```python
from build123d import *

# Parameters (mm, degrees)
SKETCH1_R                = 3.81
BOSS_EXTRUDE1_DEPTH      = 22.86
SKETCH2_R                = 3.81
BOSS_EXTRUDE2_DEPTH      = 3.81
BOSS_EXTRUDE2_DEPTH_BACK = 3.81
SKETCH4_R                = 2.54
CUT_EXTRUDE1_DEPTH       = 8.62
SKETCH5_R                = 3.302
CUT_EXTRUDE2_DEPTH       = 0.762
SKETCH6_R                = 3.302
CUT_EXTRUDE3_DEPTH       = 0.762


with BuildPart() as part:
    # Sketch1 → Boss-Extrude1 (new body)
    with BuildSketch(Plane.XY):
        with Locations((1.524, 0)):
            Circle(SKETCH1_R)
        with BuildLine():
            ThreePointArc((0, -0.762), (-0.762, 0), (0, 0.762))
            Line((0, 0.762), (0.762, 0.762))
            Line((0.762, 0.762), (0.762, 1.524))
            ThreePointArc((0.762, 1.524), (1.524, 2.286), (2.286, 1.524))
            Line((2.286, 1.524), (2.286, 0.762))
            Line((2.286, 0.762), (3.048, 0.762))
            ThreePointArc((3.048, 0.762), (3.81, 0), (3.048, -0.762))
            Line((3.048, -0.762), (2.286, -0.762))
            Line((2.286, -0.762), (2.286, -1.524))
            ThreePointArc((2.286, -1.524), (1.524, -2.286), (0.762, -1.524))
            Line((0.762, -1.524), (0.762, -0.762))
            Line((0.762, -0.762), (0, -0.762))
        make_face(mode=Mode.SUBTRACT)
    extrude(amount=BOSS_EXTRUDE1_DEPTH)

    # Sketch2 → Boss-Extrude2 (add, two sides)
    with BuildSketch(Plane(origin=(0, 0, 0), x_dir=(1, 0, 0), z_dir=(0, 1, 0))) as boss_extrude2_sk:
        with Locations((1.524, -11.43)):
            Circle(SKETCH2_R)
    extrude(amount=BOSS_EXTRUDE2_DEPTH)
    extrude(boss_extrude2_sk.sketch, amount=-BOSS_EXTRUDE2_DEPTH_BACK)

    # Sketch4 → Cut-Extrude1 (cut, through all)
    with BuildSketch(Plane(origin=(0, 3.81, 0), x_dir=(-1, 0, 0), z_dir=(0, 1, 0))):
        with Locations((-1.524, 11.43)):
            Circle(SKETCH4_R)
    extrude(amount=-CUT_EXTRUDE1_DEPTH, mode=Mode.SUBTRACT)

    # Sketch5 → Cut-Extrude2 (cut)
    with BuildSketch(Plane(origin=(0, 3.81, 0), x_dir=(1, 0, 0), z_dir=(0, 1, 0))):
        with Locations((1.524, -11.43)):
            Circle(SKETCH5_R)
    extrude(amount=-CUT_EXTRUDE2_DEPTH, mode=Mode.SUBTRACT)

    # Sketch6 → Cut-Extrude3 (cut)
    with BuildSketch(Plane.XZ.offset(3.81)):
        with Locations((1.524, 11.43)):
            Circle(SKETCH6_R)
    extrude(amount=-CUT_EXTRUDE3_DEPTH, mode=Mode.SUBTRACT)


solid = part.part
```
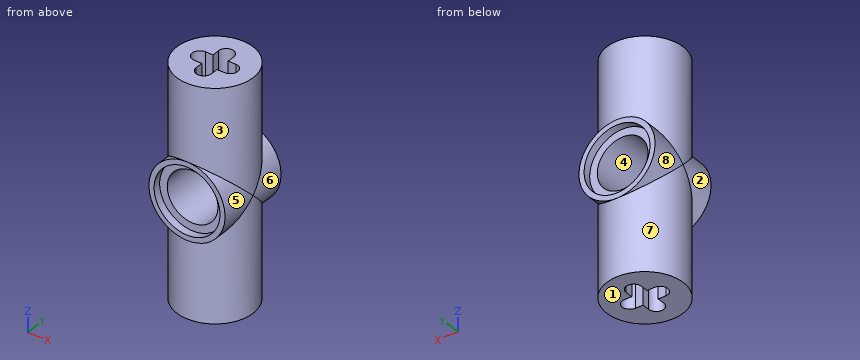
CAD build for the part. Positions are in the model's coordinates, mm. Face numbers are marked on the shaded views. A direction names the side the tool comes from. Round coordinates to 2 decimals unless told otherwise and drop trailing zeros. Loops run counter-clockwise (first coordinate to the right, second up) from the corner with the lowest first, then second, coordinate; pieces in that order, holes last. Notation, with made-up numbers: M 31.25,21 L 41.25,21 A16 cw 41.25,33 Z; hole C 84.25,5 d1. An arc over 180 degrees is marked long. Use a Markdown table: item, result. Add a question column.
(1) Drill centre lines: line 1 (Z direction, x = 0.5, y = 2.25); line 2 (Y direction, x = 3, z = 6.5); line 3 (Z direction, x = 0, y = 0.25). Where is each one in solid material? Low to high.
(2) Cut at B-B (y = 2). Give the cut face in (x, z).
(3) Cut at A-A (z = 18). Give the cut face in (x, y), and give its area (3 significant figures).
(4) Flat gauge pins, fed straight in: pin 1 (1 mm diameter, centred on y = 1, z = 8.5, fed in from +X); pin 2 (0.6 mm diameter, centred on x = 3, z = 18, fed in from -Y); pin 3 (2 mm diameter, centred on x = 0, z = 11, fed in from -Y). Where does each tip first touch, or does it go through?
(5) Cut at C-C (y = -3.5). Give the cut face in (x, z).
(6) Which spindle directions (+Z, -Z, +X, -X, +Y, -Y) get a long thin tool onto all of the face, cutting with end or side? Do the marked faces 5, 6, 7 and 8. Say none if no direction does.
(7) Pull direction Z, two halves, no side cores. Call the marked faces 1, 2, 3 and 4: +Z half, -Z half, draft (parallel to the pull), parting line (faces both ways), or undercut.
Geometry says:
| question | item | result |
|---|---|---|
| 1 | line 1 | z = 0 to 9.11, 13.75 to 22.86 |
| 1 | line 2 | y = -3.51 to -0.76, 0.76 to 3.51 |
| 1 | line 3 | z = 7.94 to 9.4, 13.46 to 14.92 |
| 2 | outline | M -1.72,0 L 0.93,0 L 0.93,7.67 A3.81 ccw 2.12,7.67 L 2.12,0 L 4.77,0 L 4.77,9.43 A3.81 ccw 4.77,13.43 L 4.77,22.86 L 2.12,22.86 L 2.12,15.19 A3.81 ccw 0.93,15.19 L 0.93,22.86 L -1.72,22.86 L -1.72,13.43 A3.81 ccw -1.72,9.43 Z; hole C 1.52,11.43 d5.08 |
| 3 | outline | C 1.52,0 d7.62; hole M 0,-0.76 L 0.76,-0.76 L 0.76,-1.52 A0.76 ccw 2.29,-1.52 L 2.29,-0.76 L 3.05,-0.76 A0.76 ccw 3.05,0.76 L 2.29,0.76 L 2.29,1.52 A0.76 ccw 0.76,1.52 L 0.76,0.76 L 0,0.76 A0.76 ccw Z |
| 3 | area | 35.0 mm² |
| 4 | pin 1 | stops at x = 5.3 |
| 4 | pin 2 | stops at y = -3.62 |
| 4 | pin 3 | stops at y = -3.05 |
| 5 | outline | M 0.02,0 L 3.03,0 L 3.03,7.93 A3.81 ccw 3.03,14.93 L 3.03,22.86 L 0.02,22.86 L 0.02,14.93 A3.81 ccw 0.02,7.93 Z; hole C 1.52,11.43 d6.6 |
| 6 | face 5 | +X, -Y |
| 6 | face 6 | +X, +Y |
| 6 | face 7 | -Z |
| 6 | face 8 | -X, +Y |
| 7 | face 1 | -Z half |
| 7 | face 2 | parting line |
| 7 | face 3 | draft |
| 7 | face 4 | undercut |
